Model file for the job. Use its own axes, mm. A direction names the side the tool comes from. Give positions to 0.01 mm unless a question says otherwise; leave off trailing zeros. Loops run counter-clockwise (first coordinate to the right, second up) from the corner with the lowest first, then second, coordinate; pieces in that order, holes last. Notation, with made-up numbers: M 51,-24.5 L 97,-24.5 A31 cw 97,5.5 Z; hole C 83.5,7.5 d4. An arc over 180 degrees is marked long. Use CSV: the item, a comma, the result in double quotes. Start each with the question number.
(1) Tool access for faces 3 (the face through (358, 129, -255.737)), 4 (the face through (35, 130, -255)), 5 (the face through (72, 140.4, -170.3)): list every direction of +Z, -Z, +X, -X, +Y, -Y with a clear straight run to the whole face (end or side of a thin tool).
(2) Slice it at C-C on y = 110. List the corners of the cut face in (x, z), and give its area (3 significant figures).
(3) Flat gauge pins, fed straight in: P1, Ø10, axis at x = 230.5, z = -220, coming from the -Y side; P2, Ø12, axis at x = 399, y = 56, coming from the -Z side; P3, Ø0.6, axis at y = -11, z = 0.5, coming from the +X side. Where does each tip first touch, or does it go through?
(4) Slice it at D-D on x = 195. List the corners of the cut face in (y, z).
(5) Wall check: line 1 along Z through (x, y) = (455, 127); line 2 along Z through (x, y) = (127, 33.5); line 3 along Y through (x, z) = (451, -93.5). Give the ranges that are in metal, low to high. Write a range as from..to.
(6) Two-plate mould, pull along X, no slides. Class faces 1 (the face through (122, 140.4, -170.3)), 2 (the face through (296, 140, -126)): pulls with the +X half, pulls with the -X half, needs draft (parallel to the pull), parting line crosses it, or undercut.
(7) Slice it at B-B on x = 466. List the corners of the cut face in (y, z), and give its area (3 significant figures).
(8) Slice it at A-A on z = -144. List the corners of the cut face in (x, y).
```python
from build123d import *

# Parameters (mm, degrees)
BASE_FLANGE1_DEPTH  = 600
SKETCH7_W           = 412
SKETCH7_H           = 20
BOSS_EXTRUDE1_DEPTH = 0.7366
SKETCH8_W           = 50
SKETCH8_H           = 170
CUT_EXTRUDE2_DEPTH  = 672.742110604


# Sheet-metal steps are written as plain solids
with BuildPart() as part:
    # Sketch1 → Base-Flange1 (new body)
    with BuildSketch(Plane(origin=(0, 0, 0), x_dir=(0, 0, -1), z_dir=(1, 0, 0))):
        with BuildLine():
            Line((0, 0), (0, 139.2634))
            ThreePointArc((0, 139.2634), (0.215745145, 139.784254855), (0.7366, 140))
            Line((0.7366, 140), (254.2634, 140))
            ThreePointArc((254.2634, 140), (254.784254855, 139.784254855), (255, 139.2634))
            Line((255, 139.2634), (255, 120))
            Line((255, 120), (255.7366, 120))
            Line((255.7366, 120), (255.7366, 139.2634))
            ThreePointArc((255.7366, 139.2634), (255.30510971, 140.30510971), (254.2634, 140.7366))
            Line((254.2634, 140.7366), (0.7366, 140.7366))
            ThreePointArc((0.7366, 140.7366), (-0.30510971, 140.30510971), (-0.7366, 139.2634))
            Line((-0.7366, 139.2634), (-0.7366, 0))
            Line((-0.7366, 0), (0, 0))
        make_face()
    extrude(amount=BASE_FLANGE1_DEPTH)

    # Sketch7 → Boss-Extrude1 (add)
    with BuildSketch(Plane.XY.offset(0.7366)):
        with Locations((206, -10)):
            Rectangle(SKETCH7_W, SKETCH7_H)
    extrude(amount=-BOSS_EXTRUDE1_DEPTH)

    # Sketch8 → Cut-Extrude2 (cut, through all)
    with BuildSketch(Plane(origin=(0, 140.7366, 0), x_dir=(1, 0, 0), z_dir=(0, 1, 0))):
        with Locations((97, 170.7366)):
            Rectangle(SKETCH8_W, SKETCH8_H)
    extrude(amount=-CUT_EXTRUDE2_DEPTH, mode=Mode.SUBTRACT)


solid = part.part
```
Reply:
1,face 3,"-Z, +X, -X, +Y, -Y"
1,face 4,"+X, -X, -Y"
1,face 5,"-Z, +Y, -Y"
2,outline,"M 0,0 L 600,0 L 600,0.74 L 0,0.74 Z"
2,area,"442 mm^2"
3,P1,"stops at y = 140"
3,P2,"stops at z = 0"
3,P3,"stops at x = 412"
4,outline,"M -20,0 L 139.26,0 A0.74 cw 140,-0.74 L 140,-254.26 A0.74 cw 139.26,-255 L 120,-255 L 120,-255.74 L 139.26,-255.74 A1.47 ccw 140.74,-254.26 L 140.74,-0.74 A1.47 ccw 139.26,0.74 L -20,0.74 Z"
5,line 1,"z = -255.74..-255, 0..0.74"
5,line 2,"z = 0..0.74"
5,line 3,"y = 140..140.74"
6,face 1,"undercut"
6,face 2,"needs draft"
7,outline,"M 0,0 L 139.26,0 A0.74 cw 140,-0.74 L 140,-254.26 A0.74 cw 139.26,-255 L 120,-255 L 120,-255.74 L 139.26,-255.74 A1.47 ccw 140.74,-254.26 L 140.74,-0.74 A1.47 ccw 139.26,0.74 L 0,0.74 Z"
7,area,"306 mm^2"
8,outline,"M 0,140 L 72,140 L 72,140.74 L 0,140.74 Z; M 122,140 L 600,140 L 600,140.74 L 122,140.74 Z"
